Check sheet for the drawn part. Datum: minimum x, y, z corner. Units: mm. Round coordinates to 2 decimals unless told otherwise and drop trailing zeros. Loops run counter-clockwise (first coordinate to the right, second up) from the corner with the lowest first, then second, coordinate; pieces in that order, holes last. Notation, with made-up numbers: (-39, 48) -> (-19, 48) arc R18 cw to (-19, 75) -> close; hole circle Ø2 at (82, 41.25). An arc over 180 degrees is marked (long way). Return JSON: item names as keys, results as strings.
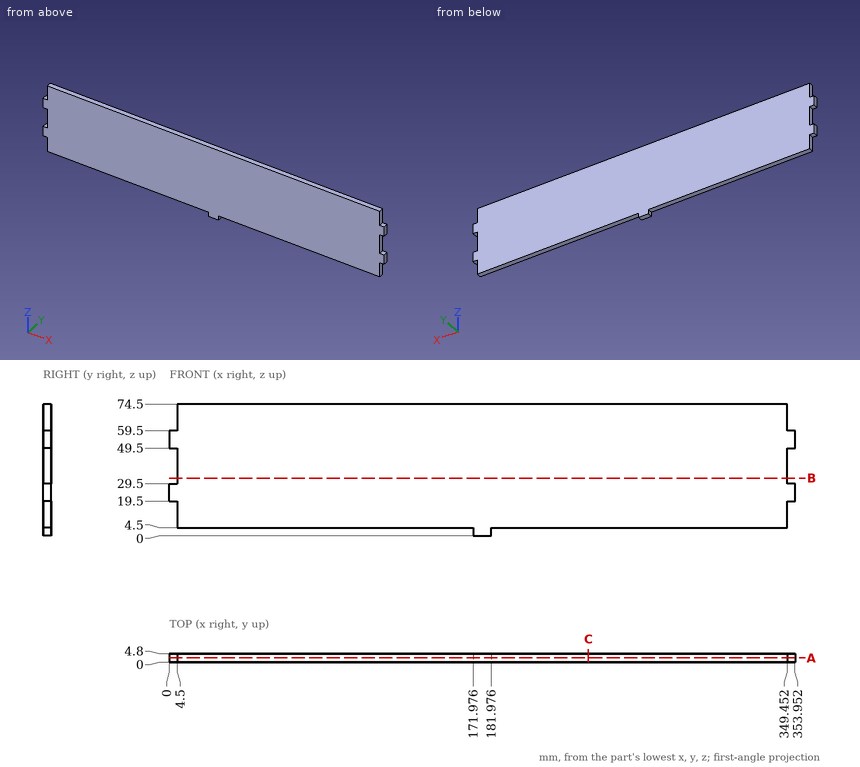
Q1. Section check B-B (z = 32.5). Record the boundary of the cut face in (x, y).
Results list:
{"outline": "(4.5, 0) -> (349.45, 0) -> (349.45, 4.8) -> (4.5, 4.8) -> close"}
Q2. Material ranges on line 1 (X direction, y = 1.25, z = 48); line 2 (Z direction, x = 139, y = 1.8), recorded low to high.
Results list:
{"line 1": "4.5 to 349.45", "line 2": "4.5 to 74.5"}
Q3. Section check A-A (y = 2.4). Record the boundary of the cut face in (x, z).
Results list:
{"outline": "(0, 19.5) -> (4.5, 19.5) -> (4.5, 4.5) -> (171.98, 4.5) -> (171.98, 0) -> (181.98, 0) -> (181.98, 4.5) -> (349.45, 4.5) -> (349.45, 19.5) -> (353.95, 19.5) -> (353.95, 29.5) -> (349.45, 29.5) -> (349.45, 49.5) -> (353.95, 49.5) -> (353.95, 59.5) -> (349.45, 59.5) -> (349.45, 74.5) -> (4.5, 74.5) -> (4.5, 59.5) -> (0, 59.5) -> (0, 49.5) -> (4.5, 49.5) -> (4.5, 29.5) -> (0, 29.5) -> close"}
Q4. Go/stop test with flat-tipped pins: pin 1 (1.4 mm diameter, centred on x = 117.5, y = 1.5, fed in from -Z); pin 2 (1.3 mm diameter, centred on x = 352.5, y = 3, fed in from -Z); pin 3 (1.4 mm diameter, centred on y = 2, z = 9, fed in from +X). Record where each tip stops, or that it passes through.
Results list:
{"pin 1": "z = 4.5", "pin 2": "z = 19.5", "pin 3": "x = 349.45"}
Q5. Section check C-C (x = 237). Record the boundary of the cut face in (y, z), then the cut area to 3 significant figures.
Results list:
{"outline": "(0, 4.5) -> (4.8, 4.5) -> (4.8, 74.5) -> (0, 74.5) -> close", "area": "336 mm^2"}
